Input: part model. Units: mm. Frame: model coordinates. A direction names the side the tool comes from. Round coordinates to 2 decimals unless told otherwise and drop trailing zeros. Loops run counter-clockwise (first coordinate to the right, second up) from the corner with the lowest first, then second, coordinate; pieces in that order, holes last.
(1) Line query: line 1 (X direction, y = -7, z = 107) (3 decimals); line 2 (Y direction, x = 2, z = 59) (3 decimals); line 3 (Y direction, x = 6.5, z = 313). Output: solid intervals per line, ascending.
(2) First-contact query: pin 1 Ø4 at (x, z) = (2, 37) entering from -Y; pin 2 Ø5 at (y, z) = (-9, 272.5) entering from -X. Flat tips, straight axial feed; report the tip coordinate or a pass-through.
(3) Access query for faces 1 (the face through (-12.7, 0, 178)), 2 (the face through (-3.175, -8, 90)), 3 (the face through (8, -8, 177.8)). Directions: +Z, -Z, +X, -X, +Y, -Y. A direction counts if a zero-diameter tool reaches every point of the face in a straight line with its end or side. Return the directions, or none.
(4) Draft query along X for faces 4 (the face through (3.175, -8, 88)), 5 (the face through (10.79, -10.89, 87.66)), 6 (the face through (8, -8, 184.15)). Return one class per face: released by +X, released by -X, zero draft, split by the parting line, or undercut.
(5) Cut plane A-A, the plane z = 86. Output: boundary loops of the cut face in (x, y) (3 decimals), and give its area (3 significant figures).
from build123d import *

# Parameters (mm, degrees)
F1_DEPTH = 361.95
F2_W     = 3.175
F2_H     = 6.35
F2_W_2   = 6.35
F3_DEPTH = 9.525
F2_H_2   = 177.8
F4_DEPTH = 9.525
F5_DEPTH = 9.525


with BuildPart() as f1:
    # F0 (on Top) → F1 (new body)
    with BuildSketch(Plane.XY):
        with BuildLine():
            ThreePointArc((12.7, 6.35), (10.8401280605, 10.8401280605), (6.35, 12.7))
            Line((6.35, 12.7), (-6.35, 12.7))
            ThreePointArc((-6.35, 12.7), (-10.8401280605, 10.8401280605), (-12.7, 6.35))
            Line((-12.7, 6.35), (-12.7, -6.35))
            ThreePointArc((-12.7, -6.35), (-10.8401280605, -10.8401280605), (-6.35, -12.7))
            Line((-6.35, -12.7), (6.35, -12.7))
            ThreePointArc((6.35, -12.7), (10.8401280605, -10.8401280605), (12.7, -6.35))
            Line((12.7, -6.35), (12.7, 6.35))
        make_face()
    extrude(amount=F1_DEPTH)

    # F2 (on face) → F3 (cut)
    with BuildSketch(Plane.XZ.offset(12.7)):
        with Locations((-4.7625, 180.975)):
            Rectangle(F2_W, F2_H)
        with Locations((-9.525, 180.975)):
            Rectangle(F2_W_2, F2_H)
        with Locations((9.525, 180.975)):
            Rectangle(F2_W_2, F2_H)
    extrude(amount=-F3_DEPTH, mode=Mode.SUBTRACT)

    # F2 (on face) → F4 (cut)
    with BuildSketch(Plane.XZ.offset(12.7)):
        with Locations((0, 273.05)):
            Rectangle(F2_W_2, F2_H_2)
        with Locations((0, 88.9)):
            Rectangle(F2_W_2, F2_H_2)
        with Locations((0, 180.975)):
            Rectangle(F2_W_2, F2_H)
    extrude(amount=-F4_DEPTH, mode=Mode.SUBTRACT)

    # F2 (on face) → F5 (cut)
    with BuildSketch(Plane.XZ.offset(12.7)):
        with Locations((4.7625, 180.975)):
            Rectangle(F2_W, F2_H)
        with Locations((9.525, 180.975)):
            Rectangle(F2_W_2, F2_H)
        with Locations((-4.7625, 180.975)):
            Rectangle(F2_W, F2_H)
        with Locations((0, 180.975)):
            Rectangle(F2_W_2, F2_H)
        with Locations((-9.525, 180.975)):
            Rectangle(F2_W_2, F2_H)
    extrude(amount=-F5_DEPTH, mode=Mode.SUBTRACT)


solid = f1.part
Reported:
1. line 1: x = -12.667 to -3.175, 3.175 to 12.667
1. line 2: y = -3.175 to 12.7
1. line 3: y = -12.7 to 12.7
2. pin 1: stops at y = -12.7
2. pin 2: stops at x = -12.7
3. face 1: +Z, -Z, -X, +Y, -Y
3. face 2: +Z, -Z, -Y
3. face 3: +X, -X, -Y
4. face 4: undercut
4. face 5: released by +X
4. face 6: zero draft
5. outline: (-12.7, -6.35) arc R6.35 ccw to (-6.35, -12.7) - (-3.175, -12.7) - (-3.175, -3.175) - (3.175, -3.175) - (3.175, -12.7) - (6.35, -12.7) arc R6.35 ccw to (12.7, -6.35) - (12.7, 6.35) arc R6.35 ccw to (6.35, 12.7) - (-6.35, 12.7) arc R6.35 ccw to (-12.7, 6.35) - close
5. area: 550 mm2
